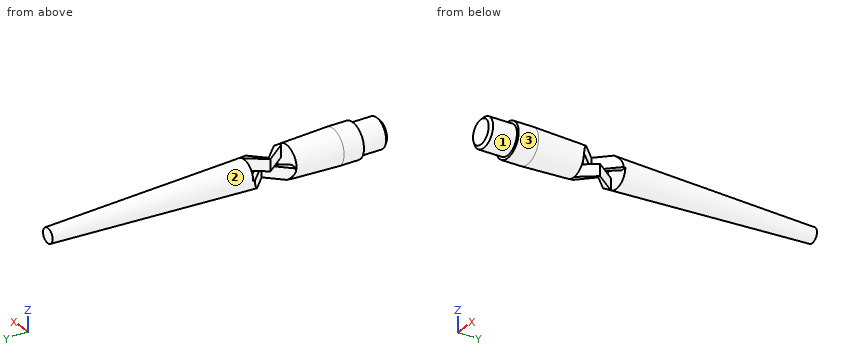
from build123d import *

# Parameters (mm, degrees)
CHAMFER1_SIZE           = 0.254
CUT_EXTRUDE1_DEPTH      = 2.54
CUT_EXTRUDE2_DEPTH      = 1.49577718
CUT_EXTRUDE3_DEPTH      = 32.835736241
CUT_EXTRUDE3_DEPTH_BACK = 32.835736241
SKETCH9_W               = 0.424246117
SKETCH9_H               = 4.064


# Read off the part's stored shape, not the designer's step: Cut-Extrude2
with BuildPart() as part:
    # Sketch1 → Revolve1 (revolve)
    with BuildSketch(Plane.XY, mode=Mode.PRIVATE) as revolve1_sk:
        Polygon((0, 0), (0, 31.75), (-0.697488389, 31.75), (-1.651, 4.445), (-1.651, 2.54), (-1.397, 2.54), (-1.397, 0), align=None)
    revolve(revolve1_sk.sketch.rotate(Axis((0, 0, 0), (0, 1, 0)), 270), axis=Axis((0, 0, 0), (0, 1, 0)))

    # Chamfer1
    chamfer1_edges = [part.edges().sort_by_distance(p)[0] for p in [
        (0, 0, 1.397),
    ]]
    chamfer(chamfer1_edges, length=CHAMFER1_SIZE)

    # Sketch7 → Cut-Extrude1 (cut)
    with BuildSketch(Plane.XY):
        Polygon((-1.778, 13.208), (0.508, 10.922), (-1.778, 8.636), align=None)
        Polygon((-0.762, 12.954), (2.54, 12.954), (2.54, 8.89), (-0.762, 8.89), (0.762, 10.922), align=None)
    extrude(amount=-CUT_EXTRUDE1_DEPTH, mode=Mode.SUBTRACT)

    # Cut-Extrude2 outline → Cut-Extrude2 (cut)
    with BuildSketch(Plane.XY):
        Polygon((-0.508, 10.922), (1.778, 8.636), (1.778, 13.208), align=None)
        Polygon((-2.54, 8.89), (0.762, 8.89), (-0.762, 10.922), (0.762, 12.954), (-2.54, 12.954), align=None)
    extrude(amount=CUT_EXTRUDE2_DEPTH, mode=Mode.SUBTRACT)

    # Sketch9 → Cut-Extrude3 (cut, two sides: drawn at the far end of the back side and taken through both)
    with BuildSketch(Plane(origin=(0, 0, 0), x_dir=(0, 0, -1), z_dir=(1, 0, 0)).offset(-CUT_EXTRUDE3_DEPTH_BACK)):
        with Locations((-1.331180992, 10.922)):
            Rectangle(SKETCH9_W, SKETCH9_H)
        with Locations((1.331180992, 10.922)):
            Rectangle(SKETCH9_W, SKETCH9_H)
    extrude(amount=CUT_EXTRUDE3_DEPTH + CUT_EXTRUDE3_DEPTH_BACK, mode=Mode.SUBTRACT)


solid = part.part
Part model, mm, in its own coordinate system. Face numbers are marked on the shaded views. A direction names the side the tool comes from. Round coordinates to 2 decimals unless told otherwise and drop trailing zeros. Loops run counter-clockwise (first coordinate to the right, second up) from the corner with the lowest first, then second, coordinate; pieces in that order, holes last. Notation, with made-up numbers: (8, -25.5) - (27, -25.5) arc R11 ccw to (27, -20.5) - close; hole circle Ø4 at (15, 37.25). An arc over 180 degrees is marked (long way). Answer as a JSON object with one key per item and string values.
Item 1: Band-saw the part on B-B on y = 23. List the corners of the cut face in (x, z), plus the area to 3 significant figures.
Output:
{"outline": "circle Ø2.01 at (0, 0)", "area": "3.16 mm2"}
Item 2: Tool access for the marked faces 1, 2 and 3: list every direction of +Z, -Z, +X, -X, +Y, -Y with a clear straight run to the whole face (end or side of a thin tool).
Output:
{"face 1": "-Y", "face 2": "+Y", "face 3": "+Y, -Y"}
Item 3: Pin check, flat tips, straight feed: pin 1 (1.5 mm diameter, centred on y = 3, z = 1, fed in from +X); pin 2 (0.7 mm diameter, centred on x = 1, y = 12, fed in from -Z); pin 3 (1.5 mm diameter, centred on y = 20.5, z = 0, fed in from +X); pin 4 (0.5 mm diameter, centred on x = 0, y = 11, fed in from +Z). Stop position of each tip, or through.
Output:
{"pin 1": "x = 1.63", "pin 2": "z = 0", "pin 3": "x = 1.12", "pin 4": "through"}
Item 4: Band-saw the part on A-A on y = 18. List the corners of the cut face in (x, z).
Output:
{"outline": "circle Ø2.36 at (0, 0)"}
Item 5: Wall check: L1, parallel to Y at x = -0.45, z = -0.25; L2, parallel to Z at x = -0.65, y = 23; L3, parallel to X at y = 7, z = -1.2. Give the ranges that are in metal, low to high.
Output:
{"L1": "0 to 8.89, 9.31 to 9.96, 11.88 to 12.54, 12.95 to 31.75", "L2": "-0.76 to 0.76", "L3": "-1 to 1"}
